from build123d import *

# Parameters (mm, degrees)
SKETCH5_W                   = 15
SKETCH5_H                   = 7.525
CUT_EXTRUDE_START           = -15
CUT_EXTRUDE_1_OUTLINE_R     = 2.5
CUT_EXTRUDE_1_DEPTH         = 15
CUT_EXTRUDE_START_2         = -21
CUT_EXTRUDE_1_2_OUTLINE_R   = 4
CUT_EXTRUDE_1_2_OUTLINE_R_2 = 2.5
CUT_EXTRUDE_1_2_DEPTH       = 6
CUT_EXTRUDE_START_3         = -14.5
CUT_EXTRUDE_1_3_DEPTH       = 14
CUT_EXTRUDE_START_4         = 1
CUT_EXTRUDE_1_5_OUTLINE_R   = 1.433256124
CUT_EXTRUDE_1_5_DEPTH       = 6.353381724


with BuildPart() as part:
    # Sketch5 → body (revolve)
    with BuildSketch(Plane(origin=(0, 0, 0), x_dir=(0, 0, -1), z_dir=(1, 0, 0)), mode=Mode.PRIVATE) as body_sk:
        with Locations((7.5, 3.7625)):
            Rectangle(SKETCH5_W, SKETCH5_H)
    revolve(body_sk.sketch.rotate(Axis((0, 0, 0), (0, 0, 1)), 270), axis=Axis((0, 0, 0), (0, 0, 1)))

    # Вырез-Вытянуть1: read off the stored shape, not the designer's step
    # Вырез-Вытянуть1 outline → Вырез-Вытянуть1 (cut)
    with BuildSketch(Plane.XY.offset(CUT_EXTRUDE_START)):
        Circle(CUT_EXTRUDE_1_OUTLINE_R)
    extrude(amount=CUT_EXTRUDE_1_DEPTH, mode=Mode.SUBTRACT)

    # Cut-Extrude 1 2 outline → Cut-Extrude 1 2 (add)
    with BuildSketch(Plane.XY.offset(CUT_EXTRUDE_START_2)):
        Circle(CUT_EXTRUDE_1_2_OUTLINE_R)
        Circle(CUT_EXTRUDE_1_2_OUTLINE_R_2, mode=Mode.SUBTRACT)
    extrude(amount=CUT_EXTRUDE_1_2_DEPTH)

    # Cut-Extrude 1 3 outline → Cut-Extrude 1 3 (cut)
    with BuildSketch(Plane.XY.offset(CUT_EXTRUDE_START_3)):
        with BuildLine():
            ThreePointArc((1.178506304, 7.090189781), (1.362296798, 7.304241747), (1.641646979, 7.343747013))
            ThreePointArc((1.641646979, 7.343747013), (0, 7.525), (-1.641646979, 7.343747013))
            ThreePointArc((-1.641646979, 7.343747013), (-1.362296798, 7.304241747), (-1.178506304, 7.090189781))
            Line((-1.178506304, 7.090189781), (-0.995794033, 6.588191943))
            ThreePointArc((-0.995794033, 6.588191943), (-0.84934756, 6.397339182), (-0.619916985, 6.325))
            Line((-0.619916985, 6.325), (0.619916985, 6.325))
            ThreePointArc((0.619916985, 6.325), (0.84934756, 6.397339182), (0.995794033, 6.588191943))
            Line((0.995794033, 6.588191943), (1.178506304, 7.090189781))
        make_face()
        with BuildLine():
            ThreePointArc((5.644666496, 4.976280253), (4.423084023, 6.087852883), (2.988425886, 6.90615202))
            ThreePointArc((2.988425886, 6.90615202), (3.191204317, 6.709993671), (3.214077361, 6.428792651))
            Line((3.214077361, 6.428792651), (3.066827768, 5.915272291))
            ThreePointArc((3.066827768, 5.915272291), (3.073125016, 5.674790087), (3.216218345, 5.481410551))
            Line((3.216218345, 5.481410551), (4.219265096, 4.752654428))
            ThreePointArc((4.219265096, 4.752654428), (4.447398235, 4.676322148), (4.678056359, 4.744646197))
            Line((4.678056359, 4.744646197), (5.120940617, 5.043375401))
            ThreePointArc((5.120940617, 5.043375401), (5.395446839, 5.108517737), (5.644666496, 4.976280253))
        make_face()
        with BuildLine():
            ThreePointArc((-3.214077361, 6.428792651), (-3.191204317, 6.709993671), (-2.988425886, 6.90615202))
            ThreePointArc((-2.988425886, 6.90615202), (-4.423084023, 6.087852883), (-5.644666496, 4.976280253))
            ThreePointArc((-5.644666496, 4.976280253), (-5.395446839, 5.108517737), (-5.120940617, 5.043375401))
            Line((-5.120940617, 5.043375401), (-4.678056359, 4.744646197))
            ThreePointArc((-4.678056359, 4.744646197), (-4.447398235, 4.676322148), (-4.219265096, 4.752654428))
            Line((-4.219265096, 4.752654428), (-3.216218345, 5.481410551))
            ThreePointArc((-3.216218345, 5.481410551), (-3.073125016, 5.674790087), (-3.066827768, 5.915272291))
            Line((-3.066827768, 5.915272291), (-3.214077361, 6.428792651))
        make_face()
        with BuildLine():
            ThreePointArc((7.491615266, 0.708043573), (7.156700285, 2.325352883), (6.477021636, 3.830641686))
            ThreePointArc((6.477021636, 3.830641686), (6.525773848, 3.552756077), (6.378992717, 3.311815235))
            Line((6.378992717, 3.311815235), (5.958025599, 2.982919676))
            ThreePointArc((5.958025599, 2.982919676), (5.821768286, 2.784664057), (5.823867582, 2.544108577))
            Line((5.823867582, 2.544108577), (6.206997349, 1.364956402))
            ThreePointArc((6.206997349, 1.364956402), (6.346693946, 1.169108995), (6.573460157, 1.088806868))
            Line((6.573460157, 1.088806868), (7.107349669, 1.070163036))
            ThreePointArc((7.107349669, 1.070163036), (7.367719572, 0.961513584), (7.491615266, 0.708043573))
        make_face()
        with BuildLine():
            ThreePointArc((-6.378992717, 3.311815235), (-6.525773848, 3.552756077), (-6.477021636, 3.830641686))
            ThreePointArc((-6.477021636, 3.830641686), (-7.156700285, 2.325352883), (-7.491615266, 0.708043573))
            ThreePointArc((-7.491615266, 0.708043573), (-7.367719572, 0.961513584), (-7.107349669, 1.070163036))
            Line((-7.107349669, 1.070163036), (-6.573460157, 1.088806868))
            ThreePointArc((-6.573460157, 1.088806868), (-6.346693946, 1.169108995), (-6.206997349, 1.364956402))
            Line((-6.206997349, 1.364956402), (-5.823867582, 2.544108577))
            ThreePointArc((-5.823867582, 2.544108577), (-5.821768286, 2.784664057), (-5.958025599, 2.982919676))
            Line((-5.958025599, 2.982919676), (-6.378992717, 3.311815235))
        make_face()
        with BuildLine():
            ThreePointArc((6.477021636, -3.830641686), (7.156700285, -2.325352883), (7.491615266, -0.708043573))
            ThreePointArc((7.491615266, -0.708043573), (7.367719572, -0.961513584), (7.107349669, -1.070163036))
            Line((7.107349669, -1.070163036), (6.573460157, -1.088806868))
            ThreePointArc((6.573460157, -1.088806868), (6.346693946, -1.169108995), (6.206997349, -1.364956402))
            Line((6.206997349, -1.364956402), (5.823867582, -2.544108577))
            ThreePointArc((5.823867582, -2.544108577), (5.821768286, -2.784664057), (5.958025599, -2.982919676))
            Line((5.958025599, -2.982919676), (6.378992717, -3.311815235))
            ThreePointArc((6.378992717, -3.311815235), (6.525773848, -3.552756077), (6.477021636, -3.830641686))
        make_face()
        with BuildLine():
            ThreePointArc((-7.107349669, -1.070163036), (-7.367719572, -0.961513584), (-7.491615266, -0.708043573))
            ThreePointArc((-7.491615266, -0.708043573), (-7.156700285, -2.325352883), (-6.477021636, -3.830641686))
            ThreePointArc((-6.477021636, -3.830641686), (-6.525773848, -3.552756077), (-6.378992717, -3.311815235))
            Line((-6.378992717, -3.311815235), (-5.958025599, -2.982919676))
            ThreePointArc((-5.958025599, -2.982919676), (-5.821768286, -2.784664057), (-5.823867582, -2.544108577))
            Line((-5.823867582, -2.544108577), (-6.206997349, -1.364956402))
            ThreePointArc((-6.206997349, -1.364956402), (-6.346693946, -1.169108995), (-6.573460157, -1.088806868))
            Line((-6.573460157, -1.088806868), (-7.107349669, -1.070163036))
        make_face()
        with BuildLine():
            ThreePointArc((2.988425886, -6.90615202), (4.423084023, -6.087852883), (5.644666496, -4.976280253))
            ThreePointArc((5.644666496, -4.976280253), (5.395446839, -5.108517737), (5.120940617, -5.043375401))
            Line((5.120940617, -5.043375401), (4.678056359, -4.744646197))
            ThreePointArc((4.678056359, -4.744646197), (4.447398235, -4.676322148), (4.219265096, -4.752654428))
            Line((4.219265096, -4.752654428), (3.216218345, -5.481410551))
            ThreePointArc((3.216218345, -5.481410551), (3.073125016, -5.674790087), (3.066827768, -5.915272291))
            Line((3.066827768, -5.915272291), (3.214077361, -6.428792651))
            ThreePointArc((3.214077361, -6.428792651), (3.191204317, -6.709993671), (2.988425886, -6.90615202))
        make_face()
        with BuildLine():
            ThreePointArc((-5.120940617, -5.043375401), (-5.395446839, -5.108517737), (-5.644666496, -4.976280253))
            ThreePointArc((-5.644666496, -4.976280253), (-4.423084023, -6.087852883), (-2.988425886, -6.90615202))
            ThreePointArc((-2.988425886, -6.90615202), (-3.191204317, -6.709993671), (-3.214077361, -6.428792651))
            Line((-3.214077361, -6.428792651), (-3.066827768, -5.915272291))
            ThreePointArc((-3.066827768, -5.915272291), (-3.073125016, -5.674790087), (-3.216218345, -5.481410551))
            Line((-3.216218345, -5.481410551), (-4.219265096, -4.752654428))
            ThreePointArc((-4.219265096, -4.752654428), (-4.447398235, -4.676322148), (-4.678056359, -4.744646197))
            Line((-4.678056359, -4.744646197), (-5.120940617, -5.043375401))
        make_face()
        with BuildLine():
            ThreePointArc((-1.641646979, -7.343747013), (0, -7.525), (1.641646979, -7.343747013))
            ThreePointArc((1.641646979, -7.343747013), (1.362296798, -7.304241747), (1.178506304, -7.090189781))
            Line((1.178506304, -7.090189781), (0.995794033, -6.588191943))
            ThreePointArc((0.995794033, -6.588191943), (0.84934756, -6.397339182), (0.619916985, -6.325))
            Line((0.619916985, -6.325), (-0.619916985, -6.325))
            ThreePointArc((-0.619916985, -6.325), (-0.84934756, -6.397339182), (-0.995794033, -6.588191943))
            Line((-0.995794033, -6.588191943), (-1.178506304, -7.090189781))
            ThreePointArc((-1.178506304, -7.090189781), (-1.362296798, -7.304241747), (-1.641646979, -7.343747013))
        make_face()
    extrude(amount=CUT_EXTRUDE_1_3_DEPTH, mode=Mode.SUBTRACT)

    # Cut-Extrude 1 4 outline → Cut-Extrude 1 4 (revolve)
    with BuildSketch(Plane.XZ):
        Polygon((7.525, 0), (7.525, -0.5), (7.658974596, -0.5), (9.75, 0.060288568), (9.616025404, 0.560288568), align=None)
        Polygon((7.658974596, -14.5), (7.525, -14.5), (7.525, -15), (9.616025404, -15.560288568), (9.75, -15.060288568), align=None)
    revolve(axis=Axis((0, 0, 0), (0, 0, 1)))

    # Cut-Extrude 1 5 outline → Cut-Extrude 1 5 (cut)
    with BuildSketch(Plane(origin=(0, 0, 0), x_dir=(1, 0, 0), z_dir=(0, 1, 0)).offset(CUT_EXTRUDE_START_4)):
        with Locations((0, 8)):
            Circle(CUT_EXTRUDE_1_5_OUTLINE_R)
    extrude(amount=CUT_EXTRUDE_1_5_DEPTH, mode=Mode.SUBTRACT)


solid = part.part
Build history of the part. All positions in model axes, mm. A direction names the side the tool comes from. Round coordinates to 2 decimals unless told otherwise and drop trailing zeros. Write each loop counter-clockwise with the first axis right and the second up, starting at its lowest first coordinate (ties: lowest second). Pieces come first, ordered by that corner, then holes. Notation, with made-up numbers: (-14, 67.25) -> (36, 67.25) arc R19 ccw to (36, 103.25) -> close; hole circle Ø9 at (36.25, -7.75). An arc over 180 degrees is marked (long way). Use one line per item in the form item = value.
Q1. Tool access for faces 1 (the flat face through (-3.4, -5.6, -0.5)), 2 (the cylindrical face through (2.32, -7.16, -7.6)), 3 (the flat face through (6, -2, -8)), 4 (the cylindrical face through (-2.32, 7.16, -7.6)), 5 (the cylindrical face through (-6.09, -4.42, -7.6)): list every direction of +Z, -Z, +X, -X, +Y, -Y with a clear straight run to the whole face (end or side of a thin tool).
Conclusion:
face_1 = none
face_2 = +X, -Y
face_3 = +X
face_4 = -X, +Y
face_5 = -X, -Y
Q2. Band-saw the part on A-A, the plane x = 0. State how many separate pieces and enclosed holes the cut face has, then the cut area to 3 significant figures.
Conclusion:
separate_pieces = 3
enclosed_holes = 0
area = 129 mm²
Q3. Band-saw the part on C-C, the plane z = -19.25. Write the cut outline in (x, y).
Conclusion:
outline = circle Ø8 at (0, 0); hole circle Ø5 at (0, 0)
Q4. Band-saw the part on B-B, the plane y = 0. Write the cut outline in (x, z) (3 decimals), then the cut area to 3 significant figures.
Conclusion:
outline = (-9.75, -15.06) -> (-9.616, -15.56) -> (-7.525, -15) -> (-4, -15) -> (-4, -21) -> (-2.5, -21) -> (-2.5, 0) -> (-7.525, 0) -> (-9.616, 0.56) -> (-9.75, 0.06) -> (-7.659, -0.5) -> (-7.525, -0.5) -> (-7.525, -14.5) -> (-7.659, -14.5) -> close; (2.5, -21) -> (4, -21) -> (4, -15) -> (7.525, -15) -> (9.616, -15.56) -> (9.75, -15.06) -> (7.659, -14.5) -> (7.525, -14.5) -> (7.525, -0.5) -> (7.659, -0.5) -> (9.75, 0.06) -> (9.616, 0.56) -> (7.525, 0) -> (2.5, 0) -> close
area = 173 mm²
Q5. Two-plate mould, pull along X, no slides. Class faces 6 (the flat face through (3.711, 5.122, -7.598)), 7 (the flat face through (-6, -2, -8)), 8 (the cylindrical face through (6.082, -4.431, -7.598)): released by +X, released by -X, zero draft, split by the parting line, or undercut.
Conclusion:
face_6 = undercut
face_7 = released by -X
face_8 = released by +X
Q6. Drill centre lines: L1, parallel to Y at x = 0, z = -18; L2, parallel to Y at x = 0, z = -10.25 (3 decimals); L3, parallel to Z at x = 0.5, y = -6.5. Where is each one in solid material? Low to high.
Conclusion:
L1 = -4 to -2.5, 2.5 to 4
L2 = -6.325 to -2.5, 2.5 to 6.325
L3 = -15 to -14.5, -0.5 to 0
Q7. Drop flat-ended pins along their axis: P1, Ø7.5, axis at x = -2.5, y = -2, coming from the +Z side; P2, Ø4, axis at x = 7.5, z = -6.5, coming from the -Y side; P3, Ø4, axis at y = 6, z = -17, coming from the -X side. Give the stop position or say it passes through.
Conclusion:
P1 = 0
P2 = -5.08
P3 = -8.44
